Here's the drawing with two shaded views (mm, measured from the low corner). I have some questions. A direction names the side the tool comes from. Coordinates: 2 decimals unless noted, no trailing zeros. Write each loop counter-clockwise with the first axis right and the second up, starting at its lowest first coordinate (ties: lowest second). Pieces come first, ordered by that corner, then holes. Notation, with made-up numbers: (89, 67) - (136, 67) arc R14 cw to (136, 94) - close; hole circle Ø11 at (80.25, 5.25). An arc over 180 degrees is marked (long way). Answer in a Markdown table with one row per item. Add a question column.
Item 1: We'd pull the mould along Z, two halves only. Please class the marked faces 1, 2 and 3: +Z half, -Z half, draft (parallel to the pull), parting line (faces both ways), or undercut.
Item 2: I'm going to push flat-ended pins straight in: pin 1 (8 mm diameter, centred on y = 5.5, z = 12.5, fed in from -X); pin 2 (5 mm diameter, centred on x = 5, z = 7, fed in from -Y); pin 3 (8 mm diameter, centred on x = 16.5, z = 5.5, fed in from -Y). Where does each tip first touch, or does it pass through?
Item 3: Imagine slicing it at C-C (z = 4.5). Please give me the cut outline in (x, y).
Item 4: If I drill on probe 1 along Z at (x, y) = (5, 17.55); probe 2 along X at (y, z) = (6.25, 10.25); probe 3 along Y at (x, z) = (10.25, 4), over which ranges is the centre line in solid material (lowest first)? Write a range as from..to.
Item 5: Which directions (+Z, -Z, +X, -X, +Y, -Y) give clear straight access to the entire face, cutting with the end or side of a thin tool? Please do the marked faces 4 and 5.
Item 6: Imagine slicing it at A-A (x = 5). Please give me the cut outline in (y, z).
Item 7: Imagine slicing it at D-D (y = 1.75). Please give me the cut outline in (x, z), plus the area to 3 significant figures.
Item 8: Imagine slicing it at B-B (z = 7.5). Please give me the cut outline in (x, y), plus the area to 3 significant figures.
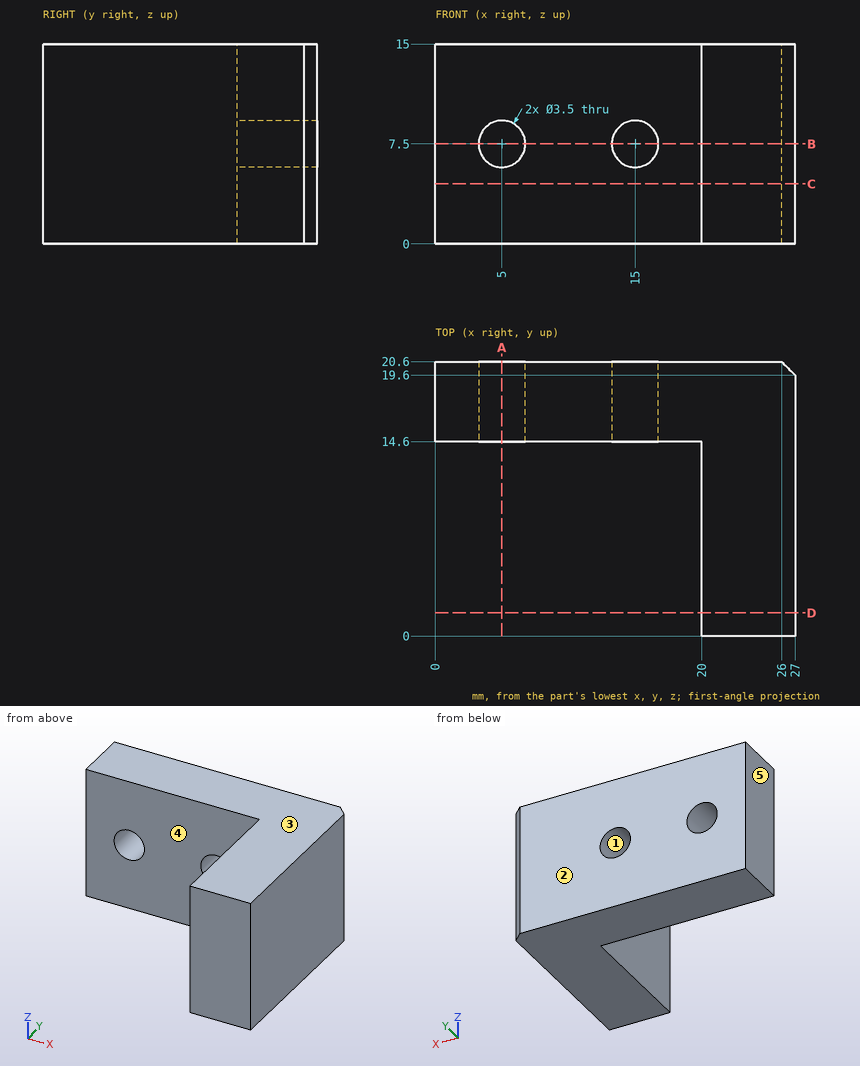
Here are the results:
| question | item | result |
|---|---|---|
| 1 | face 1 | undercut |
| 1 | face 2 | draft |
| 1 | face 3 | +Z half |
| 2 | pin 1 | stops at x = 20 |
| 2 | pin 2 | stops at y = 14.6 |
| 2 | pin 3 | stops at y = 0 |
| 3 | outline | (0, 14.6) - (20, 14.6) - (20, 0) - (27, 0) - (27, 19.6) - (26, 20.6) - (0, 20.6) - close |
| 4 | probe 1 | z = 0..5.75, 9.25..15 |
| 4 | probe 2 | x = 20..27 |
| 4 | probe 3 | y = 14.6..20.6 |
| 5 | face 4 | +Z, -Z, -X, -Y |
| 5 | face 5 | +Z, -Z, -X, +Y, -Y |
| 6 | outline | (14.6, 0) - (20.6, 0) - (20.6, 5.75) - (14.6, 5.75) - close; (14.6, 9.25) - (20.6, 9.25) - (20.6, 15) - (14.6, 15) - close |
| 7 | outline | (20, 0) - (27, 0) - (27, 15) - (20, 15) - close |
| 7 | area | 105 mm2 |
| 8 | outline | (0, 14.6) - (3.25, 14.6) - (3.25, 20.6) - (0, 20.6) - close; (6.75, 14.6) - (13.25, 14.6) - (13.25, 20.6) - (6.75, 20.6) - close; (16.75, 14.6) - (20, 14.6) - (20, 0) - (27, 0) - (27, 19.6) - (26, 20.6) - (16.75, 20.6) - close |
| 8 | area | 222 mm2 |
